Check sheet for the drawn part. Datum: minimum x, y, z corner. Units: mm. A direction names the side the tool comes from. Round coordinates to 2 decimals unless told otherwise and drop trailing zeros. Write each loop counter-clockwise with the first axis right and the second up, starting at its lowest first coordinate (ties: lowest second). Pieces come first, ordered by that corner, then holes. Notation, with made-up numbers: M 11,43.25 L 16,43.25 A20 ccw 16,49.25 Z; hole C 46.25,-37.5 d6. An arc over 180 degrees is marked long. Put each result on its own line as item: value.
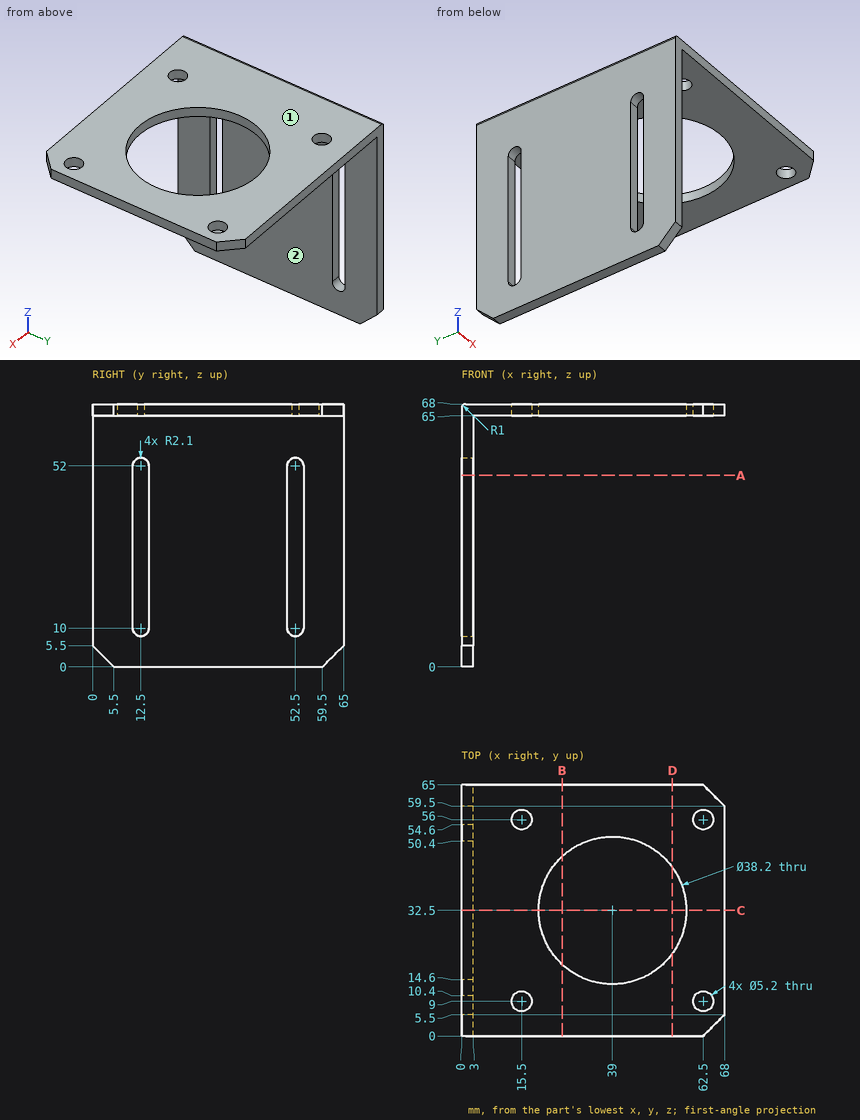
1. Depth check by flat-ended pin: pin 1 Ø1.5 at (x, z) = (2, 32) entering from -Y; pin 2 Ø6 at (x, y) = (15.5, 56) entering from -Z; pin 3 Ø4 at (y, z) = (38, 51.5) entering from +X; pin 4 Ø10 at (x, z) = (22, 59) entering from -Y. Enter the tip coordinate at first touch or a pass-through.
Computed values:
pin 1: stops at y = 0
pin 2: stops at z = 65
pin 3: stops at x = 3
pin 4: passes through
2. Cross-section at C-C (y = 32.5). Enter the section's corners in (x, z), then the cut area to 3 significant figures.
Computed values:
outline: M 0,0 L 3,0 L 3,65 L 19.9,65 L 19.9,68 L 1,68 A1 ccw 0,67 Z; M 58.1,65 L 68,65 L 68,68 L 58.1,68 Z
area: 284 mm2
3. Cross-section at D-D (x = 54.5). Enter the section's corners in (y, z), then the cut area to 3 significant figures.
Computed values:
outline: M 0,65 L 21.34,65 L 21.34,68 L 0,68 Z; M 43.66,65 L 65,65 L 65,68 L 43.66,68 Z
area: 128 mm2
4. Scan lines: probe 1 along Y at (x, z) = (15, 66); probe 2 along X at (y, z) = (53.5, 64); probe 3 along Z at (x, y) = (34, 5.5). Record each from-to range of solid material in increasing order.
Computed values:
probe 1: y = 0 to 6.45, 11.55 to 53.45, 58.55 to 65
probe 2: x = 0 to 3
probe 3: z = 65 to 68
5. Access from +Z, -Z, +X, -X, +Y, -Y to the whole of each face (thin tool, end or side, straight path). Record for the marked faces 1 and 2.
Computed values:
face 1: +Z, +X, -X, +Y, -Y
face 2: -Z, +X, +Y, -Y
6. Cross-section at B-B (x = 26). Enter the section's corners in (y, z), then the cut area to 3 significant figures.
Computed values:
outline: M 0,65 L 18.51,65 L 18.51,68 L 0,68 Z; M 46.49,65 L 65,65 L 65,68 L 46.49,68 Z
area: 111 mm2
7. Cross-section at A-A (z = 49.5). Enter the section's corners in (x, y).
Computed values:
outline: M 0,0 L 3,0 L 3,10.4 L 0,10.4 Z; M 0,14.6 L 3,14.6 L 3,50.4 L 0,50.4 Z; M 0,54.6 L 3,54.6 L 3,65 L 0,65 Z
